from build123d import *

# Parameters (mm, degrees)
F0_W      = 84.25
F0_H      = 59.75
F1_DEPTH  = 11
F2_W      = 80.25
F2_H      = 55.75
F3_DEPTH  = 9
F4_W      = 82.25
F4_H      = 57.75
F4_W_2    = 80.25
F4_H_2    = 55.75
F5_DEPTH  = 2
F6_W      = 7.5
F6_H      = 7
F7_DEPTH  = 1.25
F8_R      = 1
F9_W      = 7.5
F9_H      = 2
F10_DEPTH = 1
F11_SIZE  = 0.8


with BuildPart() as f1:
    # F0 (on Top) → F1 (new body)
    with BuildSketch(Plane.XY):
        Rectangle(F0_W, F0_H)
    extrude(amount=F1_DEPTH)

    # F2 (on face) → F3 (cut)
    with BuildSketch(Plane(origin=(0, 0, 0), x_dir=(1, 0, 0), z_dir=(0, 0, -1))):
        Rectangle(F2_W, F2_H)
    extrude(amount=-F3_DEPTH, mode=Mode.SUBTRACT)

    # F4 (on face) → F5 (cut)
    with BuildSketch(Plane(origin=(0, 0, 0), x_dir=(1, 0, 0), z_dir=(0, 0, -1))):
        Rectangle(F4_W, F4_H)
        Rectangle(F4_W_2, F4_H_2, mode=Mode.SUBTRACT)
    extrude(amount=-F5_DEPTH, mode=Mode.SUBTRACT)

    # F6 (on face) → F7 (join)
    with BuildSketch(Plane.YZ.offset(-40.125)):
        with Locations((0, -1.5)):
            Rectangle(F6_W, F6_H)
        with Locations((0, 5.5)):
            Rectangle(F6_W, F6_H)
    extrude(amount=F7_DEPTH)

    # F8
    f8_edges = [f1.edges().sort_by_distance(p)[0] for p in [
        (-42.125, -29.875, 5.5),
        (42.125, -29.875, 5.5),
        (-42.125, 29.875, 5.5),
        (42.125, 29.875, 5.5),
        (0, 29.875, 11),
        (-42.125, 0, 11),
        (0, -29.875, 11),
        (42.125, 0, 11),
    ]]
    fillet(f8_edges, radius=F8_R)

    # F9 (on face) → F10 (join)
    with BuildSketch(Plane(origin=(-40.125, 0, 0), x_dir=(0, -1, 0), z_dir=(-1, 0, 0))):
        with Locations((0, -4)):
            Rectangle(F9_W, F9_H)
    extrude(amount=F10_DEPTH)

    # F11
    f11_edges = [f1.edges().sort_by_distance(p)[0] for p in [
        (-41.125, 0, -3),
        (-41.125, 3.75, -4),
        (-41.125, 0, -5),
        (-41.125, -3.75, -4),
    ]]
    chamfer(f11_edges, length=F11_SIZE)

    # F12: F1 across plane


with BuildPart() as f1_1:
    add(f1.part)
    add(f1.part.mirror(Plane.YZ))


solid = f1_1.part
For this review, take the finished solid that the model builds, in its own axes (mm). A direction names the side the tool comes from. Give positions to 0.01 mm unless a question says otherwise; leave off trailing zeros. Order: outer loops, then holes, each group sorted by start corner. A loop starts at its lowest first (then second) coordinate and runs counter-clockwise, first axis right, second up. Notation, with made-up numbers: (31.25, -16) - (59.25, -16) arc R26 cw to (59.25, 19) - close; hole circle Ø6 at (61, 11.5). An arc over 180 degrees is marked (long way). Answer as a JSON object with one key per item and string values. Group by question number.
Item 1: Take a section at B-B on x = 3. Give the boundary of the cut face in (y, z) (3 decimals).
Item 2: Wall thickness on line 1 along X through (y, z) = (-17, 0.75) (3 decimals); line 2 along Y through (x, z) = (10, 2.5) (3 decimals); line 3 along X through (y, z) = (23, 5) (3 decimals): over which ranges is each line inside the solid? List them lowest first.
Item 3: Take a section at C-C on y = 0. Give the boundary of the cut face in (x, z) (3 decimals), and give its area (3 significant figures).
Item 4: Take a section at A-A on z = 1. Give the boundary of the cut face in (x, y) (3 decimals).
Item 5: Take a section at D-D on y = -24. Give the boundary of the cut face in (x, z) (3 decimals).
Item 6: Machinability: for faces 4 (the flat face through (-1, 27.875, 5)), 5 (the flat face through (42.125, 0, 5)), which of the approach directions +Z, -Z, +X, -X, +Y, -Y give a long, thin tool a straight path to every point of the face, cutting with its end or side? Answer none if there is none.
Item 7: Draft analysis for pull direction Z (two halves, no side actions). For faces 1 (the flat face through (40.125, 0, 0)), 2 (the flat face through (-1, 0, 11)), 3 (the flat face through (-1, 28.875, 1)), state which applies: pulls with the +Z half, pulls with the -Z half, needs draft (parallel to the pull), parting line crosses it, or undercut.
Item 8: Clearance check with flat-ended pins moving along their axes: pin 1 Ø1.5 at (y, z) = (-0.5, -1.5) entering from -X (3 decimals); pin 2 Ø1.5 at (x, y) = (29.5, -3) entering from -Z. State where each tip first meets the part, or that it passes through.
Reported:
{
 "1": {"outline": "(-29.875, 0) - (-28.875, 0) - (-28.875, 2) - (-27.875, 2) - (-27.875, 9) - (27.875, 9) - (27.875, 2) - (28.875, 2) - (28.875, 0) - (29.875, 0) - (29.875, 10) arc R1 ccw to (28.875, 11) - (-28.875, 11) arc R1 ccw to (-29.875, 10) - close"},
 "2": {"line 1": "-42.125 to -41.125, 41.125 to 42.125", "line 2": "-29.875 to -27.875, 27.875 to 29.875", "line 3": "-42.125 to -40.125, 40.125 to 42.125"},
 "3": {"outline": "(-42.125, 0) - (-41.125, 0) - (-41.125, 2) - (-40.125, 2) - (-40.125, -3) - (-40.325, -3) - (-41.125, -3.8) - (-41.125, -4.2) - (-40.325, -5) - (-38.875, -5) - (-38.875, 9) - (38.875, 9) - (38.875, -5) - (40.325, -5) - (41.125, -4.2) - (41.125, -3.8) - (40.325, -3) - (40.125, -3) - (40.125, 2) - (41.125, 2) - (41.125, 0) - (42.125, 0) - (42.125, 10) arc R1 ccw to (41.125, 11) - (-41.125, 11) arc R1 ccw to (-42.125, 10) - close", "area": "238 mm^2"},
 "4": {"outline": "(-42.125, -28.875) arc R1 ccw to (-41.125, -29.875) - (41.125, -29.875) arc R1 ccw to (42.125, -28.875) - (42.125, 28.875) arc R1 ccw to (41.125, 29.875) - (-41.125, 29.875) arc R1 ccw to (-42.125, 28.875) - close; (-40.125, -3.75) - (-38.875, -3.75) - (-38.875, 3.75) - (-40.125, 3.75) - close; (38.875, -3.75) - (40.125, -3.75) - (40.125, 3.75) - (38.875, 3.75) - close; hole (-41.125, -28.875) - (41.125, -28.875) - (41.125, 28.875) - (-41.125, 28.875) - close"},
 "5": {"outline": "(-42.125, 0) - (-41.125, 0) - (-41.125, 2) - (-40.125, 2) - (-40.125, 9) - (40.125, 9) - (40.125, 2) - (41.125, 2) - (41.125, 0) - (42.125, 0) - (42.125, 10) arc R1 ccw to (41.125, 11) - (-41.125, 11) arc R1 ccw to (-42.125, 10) - close"},
 "6": {"face 4": "-Z", "face 5": "+Z, -Z, +X, +Y, -Y"},
 "7": {"face 1": "undercut", "face 2": "pulls with the +Z half", "face 3": "needs draft"},
 "8": {"pin 1": "x = -40.125", "pin 2": "z = 9"}
}
